Geometry check sheet. Reference: drawing and pictorial views, mm from the part's lowest x, y, z. A direction names the side the tool comes from. Give positions to 0.01 mm unless a question says otherwise; leave off trailing zeros. Order: outer loops, then holes, each group sorted by start corner. A loop starts at its lowest first (then second) coordinate and runs counter-clockwise, first axis right, second up. Notation, with made-up numbers: (-29.75, 69.25) - (-19.75, 69.25) arc R12 cw to (-19.75, 87.25) - close; hole circle Ø1 at (-28.75, 27.25). An arc over 180 degrees is marked (long way). Answer in a Markdown table with one row per item.
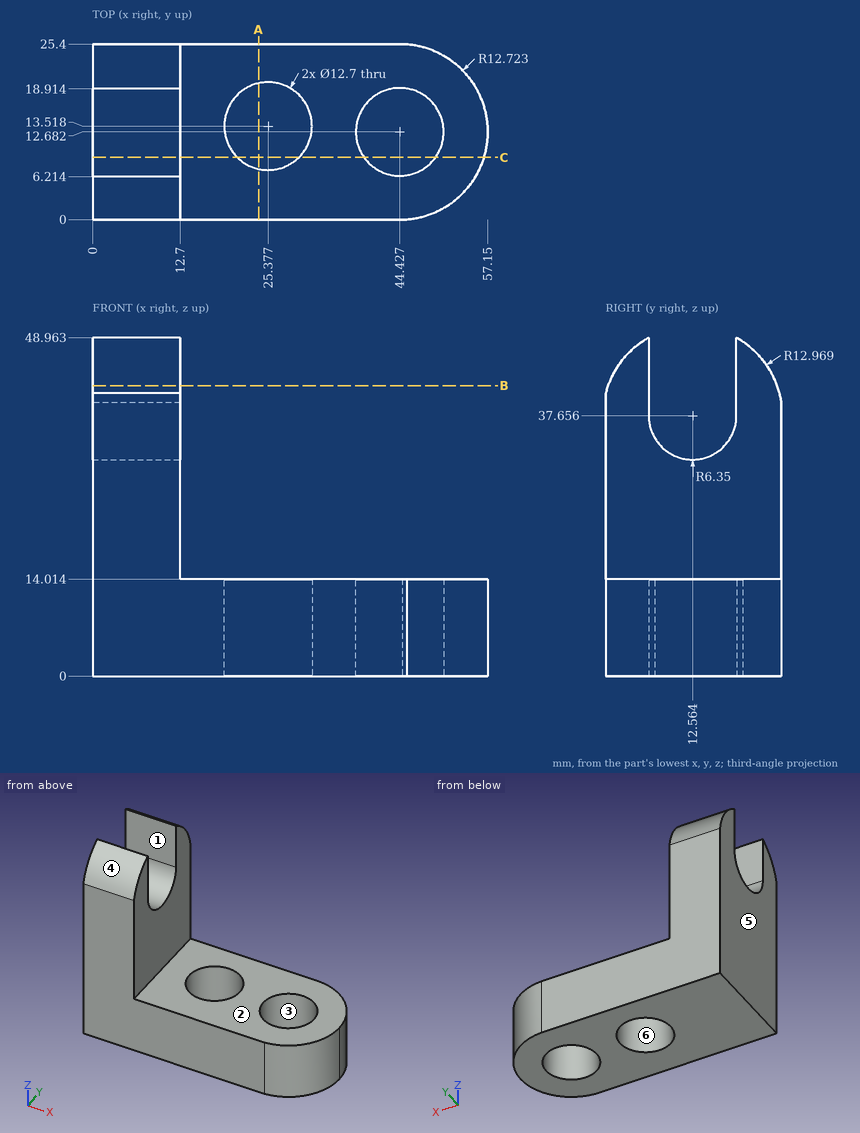
(1) Mould release check, pull along Y, two halves, no side actions. Record for the marked faces 4, 5 and 6: pulls with the +Y half, pulls with the -Y half, needs draft (parallel to the pull), parting line crosses it, or undercut.
Geometry says:
| item | result |
|---|---|
| face 4 | pulls with the -Y half |
| face 5 | needs draft |
| face 6 | undercut |
(2) Cross-section at C-C, the plane y = 9. Record the cut outline in (x, z) (1 decimal), then the cut area to 3 significant figures.
Geometry says:
| item | result |
|---|---|
| outline | (0, 0) - (20.9, 0) - (20.9, 14) - (12.7, 14) - (12.7, 32.4) - (0, 32.4) - close; (29.8, 0) - (39.3, 0) - (39.3, 14) - (29.8, 14) - close; (49.6, 0) - (56.6, 0) - (56.6, 14) - (49.6, 14) - close |
| area | 757 mm² |
(3) Cross-section at A-A, the plane x = 24. Record the cut outline in (y, z).
Geometry says:
| item | result |
|---|---|
| outline | (0, 0) - (7.32, 0) - (7.32, 14.01) - (0, 14.01) - close; (19.72, 0) - (25.4, 0) - (25.4, 14.01) - (19.72, 14.01) - close |
(4) Access from +Z, -Z, +X, -X, +Y, -Y to the whole of each face (thin tool, end or side, straight path). Record for the marked faces 1, 2 and 3.
Geometry says:
| item | result |
|---|---|
| face 1 | +Z, +X, -X |
| face 2 | +Z, +X, +Y, -Y |
| face 3 | +Z, -Z |
(5) Cross-section at B-B, the plane z = 42. Record the cut outline in (x, y) (1 decimal).
Geometry says:
| item | result |
|---|---|
| outline | (0, 0.3) - (12.7, 0.3) - (12.7, 6.2) - (0, 6.2) - close; (0, 18.9) - (12.7, 18.9) - (12.7, 24.8) - (0, 24.8) - close |
(6) Gauge pin test, flat ends, axial feed: P1, Ø12.5, axis at y = 13.5, z = 27, coming from the +X side; P2, Ø3.5, axis at x = 4.5, z = 43.5, coming from the +Y side; P3, Ø3, axis at x = 9.5, z = 40, coming from the +Y side; P4, Ø6, axis at x = 44, z = 20, coming from the -Y side. Record the tip position at first contact, or that the pin passes through.
Geometry says:
| item | result |
|---|---|
| P1 | x = 12.7 |
| P2 | y = 24.87 |
| P3 | y = 25.4 |
| P4 | through |
(7) Thickness scan on L1, parallel to X at y = 16.5, z = 19.5; L2, parallel to Y at x = 44, z = 12 (1 decimal); L3, parallel to Z at x = 37.5, y = 5.5. Record the ranges inside material, lowest first.
Geometry says:
| item | result |
|---|---|
| L1 | 0 to 12.7 |
| L2 | 0 to 6.3, 19 to 25.4 |
| L3 | 0 to 14.01 |
